For this review, take the finished solid that the model builds, in its own axes (mm). Face numbers are marked on the shaded views. A direction names the side the tool comes from. Round coordinates to 2 decimals unless told otherwise and drop trailing zeros. Write each loop counter-clockwise with the first axis right and the second up, starting at its lowest first coordinate (ties: lowest second). Pieces come first, ordered by that corner, then holes. Notation, with made-up numbers: M 88,20.25 L 105,20.25 A19 ccw 105,57.25 Z; hole C 67.5,89 d7. An arc over 180 degrees is marked long. Answer in a Markdown table with one row per item.
```python
from build123d import *

# Parameters (mm, degrees)
SKETCH_1_R               = 14
SKETCH_1_R_2             = 6
EXTRUDE_1_DEPTH          = 13
EXTRUDE_2_REACH          = 84.767
EXTRUDE_2_END_RADIUS     = 25
SKETCH_2_R               = 8
CUT_EXTRUDE_3_REACH      = 84.767
CUT_EXTRUDE_3_END_RADIUS = 14
SKETCH_3_R               = 4
FILLET_1_R               = 2


with BuildPart() as part:
    # 草圖1 → 伸長1 (new, symmetric)
    with BuildSketch(Plane(origin=(0, 0, 0), x_dir=(0, 0, -1), z_dir=(1, 0, 0))):
        with BuildLine():
            Line((-25, -33.823069051), (-25, 0))
            ThreePointArc((-25, 0), (6.428571429, 24.159335036), (21.693877551, -12.424800876))
            Line((21.693877551, -12.424800876), (4.884081633, -41.774941611))
            ThreePointArc((4.884081633, -41.774941611), (-13.114285714, -49.285043474), (-25, -33.823069051))
        make_face()
        with Locations(Location((0, 0, 0), (0, 0, 180))):
            Circle(SKETCH_1_R, mode=Mode.SUBTRACT)
        with Locations(Location((-9, -33.823069051, 0), (0, 0, 180))):
            Circle(SKETCH_1_R_2, mode=Mode.SUBTRACT)
    extrude(amount=EXTRUDE_1_DEPTH, both=True)

    # 伸長2: up to this cylinder (the profile starts outside it)
    extrude_2_end = Plane(origin=(0, 0, 0), z_dir=(-1, 0, 0)) * Cylinder(EXTRUDE_2_END_RADIUS, 220.534, mode=Mode.PRIVATE)
    # 草圖2 → 伸長2 (add, up to the surface)
    with BuildSketch(Plane(origin=(0, 28, 0), x_dir=(-1, 0, 0), z_dir=(0, 1, 0)), mode=Mode.PRIVATE) as extrude_2_sk1:
        with Locations(Location((0, 0, 0), (0, 0, 90))):
            Circle(SKETCH_2_R)
    extrude_2_tool1 = extrude(extrude_2_sk1.sketch, amount=-EXTRUDE_2_REACH, mode=Mode.PRIVATE) - extrude_2_end
    add(extrude_2_tool1.solids().sort_by_distance((0, 28, 0))[0])

    # 伸長3: up to this cylinder (the profile starts outside it)
    cut_extrude_3_end = Plane(origin=(0, 0, 0), z_dir=(-1, 0, 0)) * Cylinder(CUT_EXTRUDE_3_END_RADIUS, 198.534, mode=Mode.PRIVATE)
    # 草圖3 → 伸長3 (cut, up to the surface)
    with BuildSketch(Plane(origin=(0, 28, 0), x_dir=(1, 0, 0), z_dir=(0, 1, 0)), mode=Mode.PRIVATE) as cut_extrude_3_sk1:
        with Locations(Location((0, 0, 0), (0, 0, 270))):
            Circle(SKETCH_3_R)
    cut_extrude_3_tool1 = extrude(cut_extrude_3_sk1.sketch, amount=-CUT_EXTRUDE_3_REACH, mode=Mode.PRIVATE) - cut_extrude_3_end
    add(cut_extrude_3_tool1.solids().sort_by_distance((0, 28, 0))[0], mode=Mode.SUBTRACT)

    # 圓角1
    fillet_1_edges = [part.edges().sort_by_distance(p)[0] for p in [
        (0, 23.685438565, -8),
    ]]
    fillet(fillet_1_edges, radius=FILLET_1_R)


solid = part.part
```
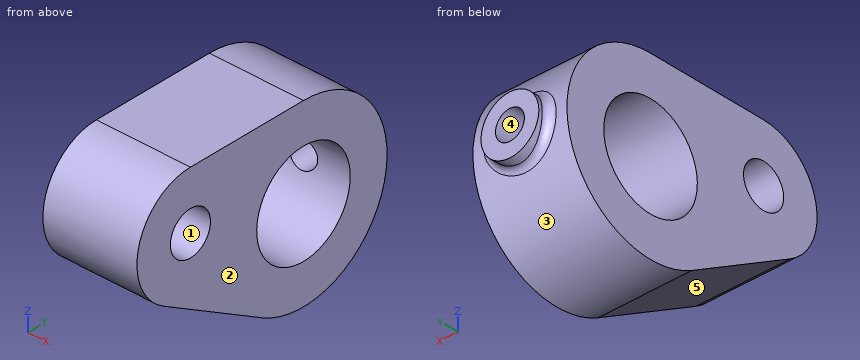
Q1. Mouldability with a two-part tool opening along Z and no side actions: class the marked faces 1, 2 and 3 as +Z half, -Z half, draft (parallel to the pull), parting line (faces both ways), or undercut.
Found:
| item | result |
|---|---|
| face 1 | undercut |
| face 2 | draft |
| face 3 | parting line |
Q2. Take a section at D-D (y = 17). State the section outline as (x, z) points.
Found:
| item | result |
|---|---|
| outline | M -13,-18.33 L 13,-18.33 L 13,18.33 L -13,18.33 Z; hole C 0,0 d8 |
Q3. Take a section at B-B (y = 6). State the section outline as (x, z) points.
Found:
| item | result |
|---|---|
| outline | M -13,-24.27 L 13,-24.27 L 13,-12.65 L -13,-12.65 Z; M -13,12.65 L 13,12.65 L 13,24.27 L -13,24.27 Z |
Q4. Take a section at A-A (y = -37.5). State the section outline as (x, z) points.
Found:
| item | result |
|---|---|
| outline | M -13,-7.33 L 13,-7.33 L 13,4.26 L -13,4.26 Z; M -13,13.74 L 13,13.74 L 13,24.57 L -13,24.57 Z |
Q5. Insertion check: P1, Ø5, axis at x = -9.5, y = 20, coming from the +Z side; P2, Ø6, axis at x = 4, z = -15, coming from the +Y side; P3, Ø12, axis at x = 4.5, y = -40, coming from the +Z side. Each pin has a flat end and moves straight along its axis. Give the tip position at first contact, or say it passes through.
Found:
| item | result |
|---|---|
| P1 | z = 17.85 |
| P2 | y = 21.93 |
| P3 | z = 25 |
Q6. Take a section at C-C (z = 0). State how many separate pieces and enclosed holes the cut face has, then the cut area to 3 significant figures.
Found:
| item | result |
|---|---|
| separate pieces | 3 |
| enclosed holes | 0 |
| area | 1,080 mm² |
Q7. For probe 1 along X at (y, z) = (22, 0); probe 2 along Z at (x, y) = (10.5, -38); probe 3 along Z at (x, y) = (11.25, -31), list the stretches that pass through material, from the lowest coordinate up.
Found:
| item | result |
|---|---|
| probe 1 | -13 to -4, 4 to 13 |
| probe 2 | -7.05 to 4.69, 13.31 to 24.45 |
| probe 3 | -11.06 to 3.71, 14.29 to 25 |
Q8. Machinability: for the marked faces 4 and 5, which of the approach directions +Z, -Z, +X, -X, +Y, -Y give a long, thin tool a straight path to every point of the face, cutting with its end or side? Answer none if there is none.
Found:
| item | result |
|---|---|
| face 4 | +Y |
| face 5 | -Z, +X, -X, -Y |
